Design review of the part built by this model. Coordinates are the model's own, in mm. A direction names the side the tool comes from. Give positions to 0.01 mm unless a question says otherwise; leave off trailing zeros. Order: outer loops, then holes, each group sorted by start corner. A loop starts at its lowest first (then second) coordinate and runs counter-clockwise, first axis right, second up. Notation, with made-up numbers: (-14, -32.75) -> (34, -32.75) arc R25 cw to (34, 1.25) -> close; hole circle Ø3 at (-19, 60). An arc over 180 degrees is marked (long way). Return JSON: item names as keys, results as strings.
```python
from build123d import *

# Parameters (mm, degrees)
SKETCH1_R           = 2.5
SKETCH1_R_2         = 1.5
BOSS_EXTRUDE1_DEPTH = 3


with BuildPart() as part:
    # Sketch1 → Boss-Extrude1 (new body)
    with BuildSketch(Plane.XY):
        with BuildLine():
            Line((-47.882351022, -2.615594916), (-50.382351022, -2.615594916))
            Line((-50.382351022, -2.615594916), (-55.382351022, -2.615594916))
            Line((-55.382351022, -2.615594916), (-70.882351022, -2.615594916))
            Line((-70.882351022, -2.615594916), (-70.882351022, 7.384405084))
            Line((-70.882351022, 7.384405084), (-55.382351022, 7.384405084))
            Line((-55.382351022, 7.384405084), (-50.382351022, 7.384405084))
            Line((-50.382351022, 7.384405084), (-47.882351022, 7.384405084))
            ThreePointArc((-47.882351022, 7.384405084), (-46.46813746, 7.970191522), (-45.882351022, 9.384405084))
            Line((-45.882351022, 9.384405084), (-45.882351022, 12))
            ThreePointArc((-45.882351022, 12), (-46.761030678, 14.121320344), (-48.882351022, 15))
            Line((-48.882351022, 15), (-67.882351022, 15))
            ThreePointArc((-67.882351022, 15), (-70.003671365, 14.121320344), (-70.882351022, 12))
            Line((-70.882351022, 12), (-70.882351022, 11.465621828))
            Line((-70.882351022, 11.465621828), (-73.882351022, 11.465621828))
            ThreePointArc((-73.882351022, 11.465621828), (-75.296564584, 10.879835391), (-75.882351022, 9.465621828))
            Line((-75.882351022, 9.465621828), (-75.882351022, -4.69681166))
            ThreePointArc((-75.882351022, -4.69681166), (-75.296564584, -6.111025222), (-73.882351022, -6.69681166))
            Line((-73.882351022, -6.69681166), (-70.882351022, -6.69681166))
            Line((-70.882351022, -6.69681166), (-70.882351022, -7))
            ThreePointArc((-70.882351022, -7), (-70.003671365, -9.121320344), (-67.882351022, -10))
            Line((-67.882351022, -10), (-48.882351022, -10))
            ThreePointArc((-48.882351022, -10), (-46.761030678, -9.121320344), (-45.882351022, -7))
            Line((-45.882351022, -7), (-45.882351022, -4.615594916))
            ThreePointArc((-45.882351022, -4.615594916), (-46.46813746, -3.201381353), (-47.882351022, -2.615594916))
        make_face()
        with Locations((-52.882351022, 10.384405084)):
            Circle(SKETCH1_R, mode=Mode.SUBTRACT)
        with Locations((-52.882351022, -5.615594916)):
            Circle(SKETCH1_R, mode=Mode.SUBTRACT)
        with Locations((-65.882351022, 10.384405084)):
            Circle(SKETCH1_R_2, mode=Mode.SUBTRACT)
        with Locations((-65.882351022, -5.615594916)):
            Circle(SKETCH1_R_2, mode=Mode.SUBTRACT)
    extrude(amount=BOSS_EXTRUDE1_DEPTH)


solid = part.part
```
Item 1: For pin 1 (6 mm diameter, centred on x = -52.88, y = 10.38, fed in from -Z); pin 2 (1.5 mm diameter, centred on x = -73, z = 1, fed in from -Y); pin 3 (0.9 mm diameter, centred on y = 3.5, z = 1.5, fed in from +X); pin 4 (0.6 mm diameter, centred on y = 11.5, z = 2, fed in from -X), all flat-tipped, find the tip position at first contact; note any pin that passes through.
Result set:
{"pin 1": "stops at z = 0", "pin 2": "stops at y = -6.7", "pin 3": "stops at x = -70.88", "pin 4": "stops at x = -74.88"}
Item 2: Add section D-D (z = 0.4). Give the boundary of the cut face in (x, y).
Result set:
{"outline": "(-75.88, -4.7) arc R2 ccw to (-73.88, -6.7) -> (-70.88, -6.7) -> (-70.88, -7) arc R3 ccw to (-67.88, -10) -> (-48.88, -10) arc R3 ccw to (-45.88, -7) -> (-45.88, -4.62) arc R2 ccw to (-47.88, -2.62) -> (-70.88, -2.62) -> (-70.88, 7.38) -> (-47.88, 7.38) arc R2 ccw to (-45.88, 9.38) -> (-45.88, 12) arc R3 ccw to (-48.88, 15) -> (-67.88, 15) arc R3 ccw to (-70.88, 12) -> (-70.88, 11.47) -> (-73.88, 11.47) arc R2 ccw to (-75.88, 9.47) -> close; hole circle Ø3 at (-65.88, -5.62); hole circle Ø3 at (-65.88, 10.38); hole circle Ø5 at (-52.88, -5.62); hole circle Ø5 at (-52.88, 10.38)"}
Item 3: Add section C-C (y = -6). Give the boundary of the cut face in (x, z).
Result set:
{"outline": "(-75.4, 0) -> (-67.33, 0) -> (-67.33, 3) -> (-75.4, 3) -> close; (-64.43, 0) -> (-55.35, 0) -> (-55.35, 3) -> (-64.43, 3) -> close; (-50.41, 0) -> (-45.88, 0) -> (-45.88, 3) -> (-50.41, 3) -> close"}
Item 4: Add section B-B (x = -52.75). Give the boundary of the cut face in (y, z), plus the area to 3 significant figures.
Result set:
{"outline": "(-10, 0) -> (-8.11, 0) -> (-8.11, 3) -> (-10, 3) -> close; (-3.12, 0) -> (-2.62, 0) -> (-2.62, 3) -> (-3.12, 3) -> close; (7.38, 0) -> (7.89, 0) -> (7.89, 3) -> (7.38, 3) -> close; (12.88, 0) -> (15, 0) -> (15, 3) -> (12.88, 3) -> close", "area": "15.0 mm^2"}
Item 5: Mouldability with a two-part tool opening along X and no side actions: class faces 1 (the face through (-64.45, 10.83, 1.48)), 2 (the face through (-58, 15, 1)), 3 (the face through (-45.882, 11, 1)) as released by +X, released by -X, zero draft, split by the parting line, or undercut.
Result set:
{"face 1": "undercut", "face 2": "zero draft", "face 3": "released by +X"}
Item 6: Add section A-A (x = -57.25). Give the boundary of the cut face in (y, z), plus the area to 3 significant figures.
Result set:
{"outline": "(-10, 0) -> (-2.62, 0) -> (-2.62, 3) -> (-10, 3) -> close; (7.38, 0) -> (15, 0) -> (15, 3) -> (7.38, 3) -> close", "area": "45.0 mm^2"}
Item 7: Wall thickness on L1, parallel to X at y = 10.75, z = 2.75; L2, parallel to Y at x = -52.5, z = 2.65 (3 decimals); L3, parallel to Y at x = -67, z = 2.8: over which ranges is each line inside the solid? List them lowest first. Write a range as [from, to].
Result set:
{"L1": "x = [-75.42, -67.34], [-64.43, -55.36], [-50.41, -45.88]", "L2": "y = [-10, -8.086], [-3.145, -2.616], [7.384, 7.914], [12.855, 15]", "L3": "y = [-10, -6.62], [-4.62, -2.62], [7.38, 9.38], [11.38, 15]"}
Item 8: Machinability: for faces 4 (the face through (-46.74, 14.1, 1.48)), 5 (the face through (-72, -6.697, 1)), 6 (the face through (-45.882, -6, 1)), 7 (the face through (-72, 11.466, 1)), 8 (the face through (-70.882, 2, 1)), which of the approach directions +Z, -Z, +X, -X, +Y, -Y give a long, thin tool a straight path to every point of the face, cutting with its end or side? Answer none if there is none.
Result set:
{"face 4": "+Z, -Z, +X, +Y", "face 5": "+Z, -Z, -X, -Y", "face 6": "+Z, -Z, +X, +Y, -Y", "face 7": "+Z, -Z, -X, +Y", "face 8": "+Z, -Z, +X"}
